CAD build for the part. Positions are in the model's coordinates, mm. A direction names the side the tool comes from. Round coordinates to 2 decimals unless told otherwise and drop trailing zeros. Order: outer loops, then holes, each group sorted by start corner. A loop starts at its lowest first (then second) coordinate and runs counter-clockwise, first axis right, second up. Notation, with made-up numbers: M 82.25,-13 L 111.25,-13 A12 cw 111.25,5 Z; hole C 43,-30 d5. An arc over 180 degrees is marked long. Answer as a JSON object with one key per item and string values.
```python
from build123d import *

# Parameters (mm, degrees)
F0_W     = 40
F0_H     = 40
F1_DEPTH = 10
F2_W     = 1.6
F2_H     = 30
F3_DEPTH = 1.25
F4_R     = 11.25
F5_DEPTH = 12.5


with BuildPart() as f1:
    # F0 (on Top) → F1 (new body)
    with BuildSketch(Plane.XY):
        Rectangle(F0_W, F0_H)
    extrude(amount=F1_DEPTH)

    # F2 (on Top) → F3 (cut, symmetric)
    with BuildSketch(Plane.XY):
        with Locations((-15, 0)):
            Rectangle(F2_W, F2_H)
        with Locations((15, 0)):
            Rectangle(F2_W, F2_H)
    extrude(amount=F3_DEPTH, both=True, mode=Mode.SUBTRACT)

    # F4 (on Top) → F5 (cut, symmetric)
    with BuildSketch(Plane.XY):
        Circle(F4_R)
    extrude(amount=F5_DEPTH, both=True, mode=Mode.SUBTRACT)


solid = f1.part
```
Item 1: Saw through at C-C on z = 6. List the corners of the cut face in (x, y), and give its area (3 significant figures).
Worked answers:
{"outline": "M -20,-20 L 20,-20 L 20,20 L -20,20 Z; hole C 0,0 d22.5", "area": "1,200 mm2"}
Item 2: Wall check: line 1 along Y through (x, z) = (0, 3.25); line 2 along X through (y, z) = (-13.5, 0.5); line 3 along Z through (x, y) = (15, 5.5). Give the ranges that are in metal, low to high. Write a range as [from, to].
Worked answers:
{"line 1": "y = [-20, -11.25], [11.25, 20]", "line 2": "x = [-20, -15.8], [-14.2, 14.2], [15.8, 20]", "line 3": "z = [1.25, 10]"}
Item 3: Drop a flat-ended pin along its axis: pin 1 Ø0.5 at (x, y) = (-15.5, 3) entering from -Z. Give the stop position or say it passes through.
Worked answers:
{"pin 1": "stops at z = 1.25"}
Item 4: Saw through at B-B on x = 1. List the corners of the cut face in (y, z), and give its area (3 significant figures).
Worked answers:
{"outline": "M -20,0 L -11.21,0 L -11.21,10 L -20,10 Z; M 11.21,0 L 20,0 L 20,10 L 11.21,10 Z", "area": "176 mm2"}
Item 5: Saw through at A-A on y = 0. List the corners of the cut face in (x, z).
Worked answers:
{"outline": "M -20,0 L -15.8,0 L -15.8,1.25 L -14.2,1.25 L -14.2,0 L -11.25,0 L -11.25,10 L -20,10 Z; M 11.25,0 L 14.2,0 L 14.2,1.25 L 15.8,1.25 L 15.8,0 L 20,0 L 20,10 L 11.25,10 Z"}
Item 6: Saw through at D-D on x = -6. List the corners of the cut face in (y, z), and give its area (3 significant figures).
Worked answers:
{"outline": "M -20,0 L -9.52,0 L -9.52,10 L -20,10 Z; M 9.52,0 L 20,0 L 20,10 L 9.52,10 Z", "area": "210 mm2"}
Item 7: Two-plate mould, pull along Y, no slides. Class faces 3 (the flat face through (-15, 0, 1.25)), 4 (the flat face through (0, 20, 5)), 5 (the flat face through (-20, 0, 5)), 6 (the flat face through (15.8, 0, 1)): released by +Y, released by -Y, zero draft, split by the parting line, or undercut.
Worked answers:
{"face 3": "undercut", "face 4": "released by +Y", "face 5": "zero draft", "face 6": "undercut"}
Item 8: 3-axis set-ups, long thin cutter, end or side, ignore diameter. For faces 1 (the flat face through (-15, -15, 1)), 2 (the flat face through (0, -20, 5)): which of +Z, -Z, +X, -X, +Y, -Y reach the whole face in a straight line?
Worked answers:
{"face 1": "-Z", "face 2": "+Z, -Z, +X, -X, -Y"}
